Geometry check sheet. Reference: the model listing, model coordinates, mm. A direction names the side the tool comes from. Give positions to 0.01 mm unless a question says otherwise; leave off trailing zeros. Order: outer loops, then holes, each group sorted by start corner. A loop starts at its lowest first (then second) coordinate and runs counter-clockwise, first axis right, second up. Notation, with made-up numbers: M -19.75,0.25 L -0.75,0.25 A22 ccw -0.75,17.25 Z; hole C 17,-18 d11. An arc over 180 degrees is marked long. Answer as a JSON object with one key per item and string values. Group by question number.
from build123d import *

# Parameters (mm, degrees)
BOSS_EXTRUDE3_DEPTH     = 12.5
SKETCH2_R               = 2.5
CUT_EXTRUDE3_DEPTH      = 4
SKETCH3_R               = 14.238624177
CUT_EXTRUDE4_DEPTH      = 26
CUT_EXTRUDE4_DEPTH_BACK = 26


with BuildPart() as part:
    # Sketch1 → Boss-Extrude3 (new body, symmetric)
    with BuildSketch(Plane(origin=(0, 0, 0), x_dir=(0, 0, -1), z_dir=(1, 0, 0))):
        with BuildLine():
            Line((0, 22), (0, -22))
            ThreePointArc((0, -22), (0.878679656, -24.121320344), (3, -25))
            Line((3, -25), (15, -25))
            Line((15, -25), (15, -21))
            Line((15, -21), (6, -21))
            ThreePointArc((6, -21), (4.585786438, -20.414213562), (4, -19))
            Line((4, -19), (4, 19))
            ThreePointArc((4, 19), (4.585786438, 20.414213562), (6, 21))
            Line((6, 21), (15, 21))
            Line((15, 21), (15, 25))
            Line((15, 25), (3, 25))
            ThreePointArc((3, 25), (0.878679656, 24.121320344), (0, 22))
        make_face()
    extrude(amount=BOSS_EXTRUDE3_DEPTH, both=True)

    # Sketch2 → Cut-Extrude3 (cut)
    with BuildSketch(Plane.XY):
        with Locations((0, 15)):
            Circle(SKETCH2_R)
        with Locations((0, -15)):
            Circle(SKETCH2_R)
    extrude(amount=-CUT_EXTRUDE3_DEPTH, mode=Mode.SUBTRACT)

    # Sketch3 → Cut-Extrude4 (cut, two sides)
    with BuildSketch(Plane(origin=(0, 0, 0), x_dir=(1, 0, 0), z_dir=(0, 1, 0))) as cut_extrude4_sk:
        with Locations((0, 25)):
            Circle(SKETCH3_R)
    extrude(amount=CUT_EXTRUDE4_DEPTH, mode=Mode.SUBTRACT)
    extrude(cut_extrude4_sk.sketch, amount=-CUT_EXTRUDE4_DEPTH_BACK, mode=Mode.SUBTRACT)


solid = part.part
1. Cross-section at B-B (z = -7.75). Record the cut outline in (x, y).
2. Access from +Z, -Z, +X, -X, +Y, -Y to the whole of each face (thin tool, end or side, straight path). Record for faces 4 (the flat face through (0, 0, -4)), 5 (the cylindrical face through (-0.158, 22.972, -10.762)).
3. Thickness scan on line 1 along Y through (x, z) = (0, -2.8); line 2 along Y through (x, z) = (0, -1.9); line 3 along Y through (x, z) = (6.75, -7.5). Record the ranges inside material, lowest first. Write a range as [from, to].
4. Release check for a two-part mould opening along Y. For faces 1 (the cylindrical face through (0.18, 20.4, -4.57)), 2 (the flat face through (0, 25, -8)), 3 (the flat face through (11, 23, -15)) record: released by +Y, released by -Y, zero draft, split by the parting line, or undercut.
5. Depth check by flat-ended pin: pin 1 (1.5 mm diameter, centred on x = 8, y = -12, fed in from -Z). Enter the tip coordinate at first touch or a pass-through.
6. Cross-section at C-C (x = 0). Record the cut outline in (y, z), and give its area (3 significant figures).
7. Cross-section at A-A (y = -15). Record the cut outline in (x, z).
8. Cross-section at D-D (x = 9). Record the cut outline in (y, z).
Report:
{
 "1": {"outline": "M -12.5,-25 L 12.5,-25 L 12.5,-21 L -12.5,-21 Z; M -12.5,21 L 12.5,21 L 12.5,25 L -12.5,25 Z"},
 "2": {"face 4": "-Z, +X, -X", "face 5": "-Z, +Y, -Y"},
 "3": {"line 1": "y = [-24.99, -17.5], [-12.5, 12.5], [17.5, 24.99]", "line 2": "y = [-24.79, -17.5], [-12.5, 12.5], [17.5, 24.79]", "line 3": "y = [-25, -21], [21, 25]"},
 "4": {"face 1": "undercut", "face 2": "released by +Y", "face 3": "zero draft"},
 "5": {"pin 1": "stops at z = -4"},
 "6": {"outline": "M -25,-10.76 L -21,-10.76 L -21,-6 A2 cw -19,-4 L -17.5,-4 L -17.5,0 L -22,0 A3 ccw -25,-3 Z; M -12.5,-4 L 12.5,-4 L 12.5,0 L -12.5,0 Z; M 17.5,-4 L 19,-4 A2 cw 21,-6 L 21,-10.76 L 25,-10.76 L 25,-3 A3 ccw 22,0 L 17.5,0 Z", "area": "212 mm2"},
 "7": {"outline": "M -12.5,-4 L -2.5,-4 L -2.5,0 L -12.5,0 Z; M 2.5,-4 L 12.5,-4 L 12.5,0 L 2.5,0 Z"},
 "8": {"outline": "M -25,-13.97 L -21,-13.97 L -21,-6 A2 cw -19,-4 L 19,-4 A2 cw 21,-6 L 21,-13.97 L 25,-13.97 L 25,-3 A3 ccw 22,0 L -22,0 A3 ccw -25,-3 Z"}
}
